```python
from build123d import *

# Parameters (mm, degrees)
SKETCH1_W                   = 38.1
SKETCH1_H                   = 38.1
SKETCH1_R                   = 4
BOSS_EXTRUDE1_DEPTH         = 5.08
F_1_4_0_25_DIAMETER_HOLE1_D = 6.35
SKETCH5_R                   = 7
SKETCH5_R_2                 = 4
BOSS_EXTRUDE2_DEPTH         = 7.92
FILLET1_R                   = 2.54
CHAMFER1_SIZE               = 1
FILLET2_R                   = 6.35


with BuildPart() as part:
    # Sketch1 → Boss-Extrude1 (new body)
    with BuildSketch(Plane(origin=(0, 0, 0), x_dir=(1, 0, 0), z_dir=(0, 1, 0))):
        Rectangle(SKETCH1_W, SKETCH1_H)
        Circle(SKETCH1_R, mode=Mode.SUBTRACT)
    extrude(amount=BOSS_EXTRUDE1_DEPTH)

    # 1/4 (0.25) Diameter Hole1 (through all)
    with Locations(Plane(origin=(0, 5.08, 0), x_dir=(1, 0, 0), z_dir=(0, 1, 0))):
        with Locations((-12.7, 12.7), (12.7, 12.7), (12.7, -12.7), (-12.7, -12.7)):
            Hole(F_1_4_0_25_DIAMETER_HOLE1_D / 2)

    # Sketch5 → Boss-Extrude2 (add)
    with BuildSketch(Plane(origin=(0, 5.08, 0), x_dir=(1, 0, 0), z_dir=(0, 1, 0))):
        Circle(SKETCH5_R)
        Circle(SKETCH5_R_2, mode=Mode.SUBTRACT)
    extrude(amount=BOSS_EXTRUDE2_DEPTH)

    # Fillet1
    fillet1_edges = [part.edges().sort_by_distance(p)[0] for p in [
        (-7, 5.08, 0),
    ]]
    fillet(fillet1_edges, radius=FILLET1_R)

    # Chamfer1
    chamfer1_edges = [part.edges().sort_by_distance(p)[0] for p in [
        (-7, 13, 0),
    ]]
    chamfer(chamfer1_edges, length=CHAMFER1_SIZE)

    # Fillet2
    fillet2_edges = [part.edges().sort_by_distance(p)[0] for p in [
        (19.05, 2.54, 19.05),
        (-19.05, 2.54, 19.05),
        (-19.05, 2.54, -19.05),
        (19.05, 2.54, -19.05),
    ]]
    fillet(fillet2_edges, radius=FILLET2_R)


solid = part.part
```
Could you check a few things on this model? Use its own coordinates, in mm. A direction names the side the tool comes from. Give positions to 0.01 mm unless a question says otherwise; leave off trailing zeros. Loops run counter-clockwise (first coordinate to the right, second up) from the corner with the lowest first, then second, coordinate; pieces in that order, holes last. Notation, with made-up numbers: (58.5, -35) - (90.5, -35) arc R26 cw to (90.5, -9) - close; hole circle Ø3 at (49.25, 47). An arc over 180 degrees is marked (long way). Answer in a Markdown table with one row per item. Add a question column.
Q1. We'd pull the mould along Z, two halves only. Please class faces 1 (the face through (-19.05, 3, 0)), 2 (the face through (11.2, 2.5, -9.9)), 3 (the face through (-17.24, 2.58, -17.14)): +Z half, -Z half, draft (parallel to the pull), parting line (faces both ways), or undercut.
Q2. If we section it at A-A (x = 0): List the corners of the cut face in (y, z) for me.
Q3. For pin 1 (5.5 mm diameter, centred on x = -12.7, z = -12.7, fed in from +Y); pin 2 (2 mm diameter, centred on y = 7, z = 1.5, fed in from +X); pin 3 (10 mm diameter, centred on x = 12.7, z = -12.7, fed in from +Y); pin 4 (4 mm diameter, centred on x = -6, y = 8.5, fed in from +Z), each with a flat end and sliding along its axis, tell me the tip position at first contact or that it passes through.
Q4. If we section it at D-D (x = 10.5): List the corners of the cut face in (y, z) for me, plus the area to 3 significant figures.
Q5. If we section it at C-C (z = 0): List the corners of the cut face in (x, y) for me, plus the area to 3 significant figures.
Q6. Please list where these lines run through material, in increasing order: L1, parallel to X at y = 3.8, z = -12.7 (3 decimals); L2, parallel to X at y = 0.75, z = -11.5. Write a range as from..to.
Q7. If we section it at B-B (y = 4.5): List the corners of the cut face in (x, z) for me (3 decimals), plus the area to 3 significant figures.
Q8. Which directions (+Z, -Z, +X, -X, +Y, -Y) give clear straight access to the entire face, cutting with the end or side of a thin tool? Please do faces 4 (the face through (-1.42, 13, 3.92)), 5 (the face through (6.466, 9.779, 2.681)).
The answers:
| question | item | result |
|---|---|---|
| 1 | face 1 | draft |
| 1 | face 2 | undercut |
| 1 | face 3 | -Z half |
| 2 | outline | (0, -19.05) - (5.08, -19.05) - (5.08, -9.54) arc R2.54 cw to (7.62, -7) - (12, -7) - (13, -6) - (13, -4) - (0, -4) - close; (0, 4) - (13, 4) - (13, 6) - (12, 7) - (7.62, 7) arc R2.54 cw to (5.08, 9.54) - (5.08, 19.05) - (0, 19.05) - close |
| 3 | pin 1 | passes through |
| 3 | pin 2 | stops at x = 7.45 |
| 3 | pin 3 | stops at y = 5.08 |
| 3 | pin 4 | stops at z = 5.74 |
| 4 | outline | (0, -19.05) - (5.08, -19.05) - (5.08, -14.99) - (0, -14.99) - close; (0, -10.41) - (5.08, -10.41) - (5.08, 10.41) - (0, 10.41) - close; (0, 14.99) - (5.08, 14.99) - (5.08, 19.05) - (0, 19.05) - close |
| 4 | area | 147 mm^2 |
| 5 | outline | (-19.05, 0) - (-4, 0) - (-4, 13) - (-6, 13) - (-7, 12) - (-7, 7.62) arc R2.54 cw to (-9.54, 5.08) - (-19.05, 5.08) - close; (4, 0) - (19.05, 0) - (19.05, 5.08) - (9.54, 5.08) arc R2.54 cw to (7, 7.62) - (7, 12) - (6, 13) - (4, 13) - close |
| 5 | area | 202 mm^2 |
| 6 | L1 | x = -19.05..-15.875, -9.525..9.525, 15.875..19.05 |
| 6 | L2 | x = -19.05..-15.64, -9.76..9.76, 15.64..19.05 |
| 7 | outline | (-19.05, -12.7) arc R6.35 ccw to (-12.7, -19.05) - (12.7, -19.05) arc R6.35 ccw to (19.05, -12.7) - (19.05, 12.7) arc R6.35 ccw to (12.7, 19.05) - (-12.7, 19.05) arc R6.35 ccw to (-19.05, 12.7) - close; hole circle Ø6.35 at (-12.7, -12.7); hole circle Ø6.35 at (-12.7, 12.7); hole circle Ø8 at (0, 0); hole circle Ø6.35 at (12.7, -12.7); hole circle Ø6.35 at (12.7, 12.7) |
| 7 | area | 1,240 mm^2 |
| 8 | face 4 | +Z, -Z, +X, -X, +Y |
| 8 | face 5 | +Y |
